from build123d import *

# Parameters (mm, degrees)
SKETCH1_W      = 35.2806
SKETCH1_H      = 39.0906
EXTRUDE1_DEPTH = 9.525
SKETCH2_R      = 7.0231
EXTRUDE2_DEPTH = 33.497714322
EXTRUDE4_DEPTH = 42.442310667
CHAMFER1_SIZE  = 2.54


with BuildPart() as part:
    # Sketch1 → Extrude1 (new, symmetric)
    with BuildSketch(Plane.XY):
        Rectangle(SKETCH1_W, SKETCH1_H)
    extrude(amount=EXTRUDE1_DEPTH, both=True)

    # Sketch2 → Extrude2 (cut, through all)
    with BuildSketch(Plane.XY.offset(9.525)):
        Circle(SKETCH2_R)
    extrude(amount=-EXTRUDE2_DEPTH, mode=Mode.SUBTRACT)

    # Sketch3 → Extrude4 (cut, through all)
    with BuildSketch(Plane.ZY.offset(17.6403)):
        Polygon((-9.525, 17.6403), (3.81, 17.6403), (3.81, -17.6403), (-9.525, -17.6403), (-9.525, 0), align=None)
    extrude(amount=-EXTRUDE4_DEPTH, mode=Mode.SUBTRACT)

    # Sketch5 → 1/8 (0.125) Diameter Hole1 (revolve, cut)
    with BuildSketch(Plane(origin=(-17.6403, 0, 6.6675), x_dir=(0, 0, 1), z_dir=(0, 1, 0))):
        Polygon((0, 0), (0, 7.303866233), (1.5875, 6.35), (1.5875, 0), align=None)
    f_1_8_0_125_diameter_hole1 = revolve(axis=Axis((-23.9903, 0, 6.6675), (1, 0, 0)), mode=Mode.SUBTRACT)

    # Mirror1: 1/8 (0.125) Diameter Hole1 across plane
    add(f_1_8_0_125_diameter_hole1.mirror(Plane(origin=(0, 0, 0), x_dir=(0, 0, 1), z_dir=(1, 0, 0))), mode=Mode.SUBTRACT)

    # Chamfer1
    chamfer1_edges = [part.edges().sort_by_distance(p)[0] for p in [
        (0, -19.5453, 9.525),
        (0, 19.5453, 9.525),
    ]]
    chamfer(chamfer1_edges, length=CHAMFER1_SIZE)


solid = part.part
Work out the finished part from the listing and answer in its coordinate system (mm). A direction names the side the tool comes from. Coordinates: 2 decimals unless noted, no trailing zeros. Loops run counter-clockwise (first coordinate to the right, second up) from the corner with the lowest first, then second, coordinate; pieces in that order, holes last. Notation, with made-up numbers: M 49.25,72 L 77.25,72 A23 cw 77.25,104 Z; hole C 89.5,-3.5 d3. An arc over 180 degrees is marked long. Answer in a Markdown table with one row per item. Add a question column.
1. A tool of negligible diameter and unlimited length cuts with its end or side. For faces 1 (the cylindrical face through (14.51, -1.073, 5.497)), 2 (the flat face through (0, -17.64, -3)), 3 (the flat face through (0, 19.545, -1)), 4 (the cylindrical face through (-14.51, -1.073, 5.497)), 5 (the cylindrical face through (6.488, -2.69, 6.708)), from which of +Z, -Z, +X, -X, +Y, -Y can it reach the whole face along a straight path? Write none if from no direction.
2. Flat-ended cylindrical pins translate along their axes: P1, Ø3, axis at x = -12.5, y = 7, coming from the -Z side; P2, Ø1.9, axis at y = 0, z = 6.67, coming from the +X side; P3, Ø4, axis at y = 0, z = 6.67, coming from the -X side. Find the tip coordinate at first contact, or state that the pin passes through.
3. Find section C-C, the plane x = -14. Write down the section's boundary in (y, z) (1 decimal).
4. The mould has two halves that part along Y. Classify faces 6 (the flat face through (0, -19, -9.525)), 7 (the flat face through (-0.25, 18.29, 8.24)), 8 (the conical face through (-10.5, -0.08, 6.93)): pulls with the +Y half, pulls with the -Y half, needs draft (parallel to the pull), parting line crosses it, or undercut.
5. Find section D-D, the plane y = -4. Write down the section's boundary in (x, z) (3 decimals).
6. Find section B-B, the plane x = 0. Write down the section's boundary in (y, z) (3 decimals), then the cut area to 3 significant figures.
7. Find section A-A, the plane z = 1.5. Write down the section's boundary in (x, y), then the cut area to 3 significant figures.
8. Consider L1, parallel to Y at x = 4, z = 3.75; L2, parallel to Y at x = 0, z = 6.45; L3, parallel to Z at x = -14.75, y = 0 (3 decimals). Determine where each line is inside the solid, lowest interval first.
Reported:
| question | item | result |
|---|---|---|
| 1 | face 1 | +X |
| 1 | face 2 | -Z, +X, -X |
| 1 | face 3 | +Z, -Z, +X, -X, +Y |
| 1 | face 4 | -X |
| 1 | face 5 | +Z, -Z |
| 2 | P1 | stops at z = 3.81 |
| 2 | P2 | stops at x = 10.91 |
| 2 | P3 | stops at x = -17.64 |
| 3 | outline | M -19.5,-9.5 L -17.6,-9.5 L -17.6,3.8 L 17.6,3.8 L 17.6,-9.5 L 19.5,-9.5 L 19.5,7 L 17,9.5 L -17,9.5 L -19.5,7 Z; hole C 0,6.7 d3.2 |
| 4 | face 6 | needs draft |
| 4 | face 7 | pulls with the +Y half |
| 4 | face 8 | undercut |
| 5 | outline | M -17.64,3.81 L -5.773,3.81 L -5.773,9.525 L -17.64,9.525 Z; M 5.773,3.81 L 17.64,3.81 L 17.64,9.525 L 5.773,9.525 Z |
| 6 | outline | M -19.545,-9.525 L -17.64,-9.525 L -17.64,3.81 L -7.023,3.81 L -7.023,9.525 L -17.005,9.525 L -19.545,6.985 Z; M 7.023,3.81 L 17.64,3.81 L 17.64,-9.525 L 19.545,-9.525 L 19.545,6.985 L 17.005,9.525 L 7.023,9.525 Z |
| 6 | area | 187 mm^2 |
| 7 | outline | M -17.64,-19.55 L 17.64,-19.55 L 17.64,-17.64 L -17.64,-17.64 Z; M -17.64,17.64 L 17.64,17.64 L 17.64,19.55 L -17.64,19.55 Z |
| 7 | area | 134 mm^2 |
| 8 | L1 | y = -19.55 to -17.64, 17.64 to 19.55 |
| 8 | L2 | y = -19.55 to -7.02, 7.02 to 19.55 |
| 8 | L3 | z = 3.81 to 5.08, 8.255 to 9.525 |
